Autodesk Inventor part; units mm, degrees
ref_plane "YZ Plane" through (0, 0, 0) normal (1, 0, 0) x (0, 1, 0)
ref_plane "XZ Plane" through (0, 0, 0) normal (0, 1, 0) x (-1, 0, 0)
ref_plane "XY Plane" through (0, 0, 0) normal (0, 0, 1) x (1, 0, 0)
sketch "スケッチ1" plane through (0, 0, 0) normal (0, 0, 1) x (1, 0, 0)
  line L0 (0, 0) -> (-10, 0)
  line L1 (-10, 0) -> (-10, -20)
  line L2 (-10, -20) -> (0, -20)
  line L3 (0, -20) -> (0, 0)
  line L4 (0, 0) -> (-35, 0)
  line L5 (-35, 0) -> (-35, 10)
  line L6 (-35, 10) -> (0, 10)
  line L7 (0, 10) -> (0, 0)
  line L8 (-5, -20) -> (-5, 0)
  line L9 (0, 5) -> (-35, 5)
  circle A0 centre (-10, 5) radius 1.6
  circle A1 centre (-5, -5) radius 1.6
  circle A2 centre (-20, 5) radius 1.6
  circle A3 centre (-30, 5) radius 1.6
  circle A4 centre (-5, -15) radius 1.6
  circle A5 centre (-5, -25) radius 1.6
  dimension "d0" = 10
  dimension "d1" = 20
  dimension "d2" = 35
  dimension "d3" = 10
  dimension "d4" = 3.2
  dimension "d5" = 3.2
  dimension "d6" = 10
  dimension "d7" = 5
  dimension "d11" = 10
  dimension "d18" = 10
extrude "押し出し1" add sketch "スケッチ1" along normal blind 2 contours L3 L2 L8 A4 A1 L0 | L0 L4 L5 L9 A3 A2 A0 L7 | L8 A1 A4 L2 L1 L0 | L9 A0 A2 A3 L5 L6 L7 | A0 L9 | L9 A0
fillet "フィレット1" radius 5 6 edges at (0, 10, 1) (-35, 10, 1) (-35, 0, 1) (0, -20, 1) (-10, -20, 1) (-10, 0, 1)
properties part number "kakutome_nc"
Work out the finished part from the listing and answer in its coordinate system (mm). A direction names the side the tool comes from. Give positions to 0.01 mm unless a question says otherwise; leave off trailing zeros. Loops run counter-clockwise (first coordinate to the right, second up) from the corner with the lowest first, then second, coordinate; pieces in that order, holes last. Notation, with made-up numbers: (-14, 38.5) -> (18, 38.5) arc R22 ccw to (18, 46.5) -> close; hole circle Ø10 at (45, 86.25). An arc over 180 degrees is marked (long way). Use a Markdown table: item, result. Add a question column.
1. Determine the mould class of faces 1 (the flat face through (-14, 2, 2)), 2 (the cylindrical face through (-5.208, -16.586, 0.986)), 3 (the flat face through (-10, -10, 1)) for opening direction X: released by +X, released by -X, zero draft, split by the parting line, or undercut.
2. Section A-A on x = -20 is taken. Determine the outline of the cut face in (y, z).
3. Section D-D on x = -16 is taken. Determine the outline of the cut face in (y, z).
4. Flat-ended cylindrical pins translate along their axes: pin 1 Ø3 at (x, y) = (-5, -5) entering from -Z; pin 2 Ø5 at (x, y) = (-5, -15) entering from -Z; pin 3 Ø1 at (y, z) = (-5.5, 0.5) entering from -X; pin 4 Ø0.6 at (x, z) = (-20.5, 1.5) entering from -Y. Find the tip coordinate at first contact, or state that the pin passes through.
5. Section C-C on y = -12.25 is taken. Determine the outline of the cut face in (x, z).
6. Section B-B on z = 1.5 is taken. State how many separate pieces and enclosed holes the cut face has, and give its area (3 significant figures).
7. For faces 4 (the flat face through (-22, 0, 1)), 5 (the cylindrical face through (-1, 8, 1)), determine the directions among +Z, -Z, +X, -X, +Y, -Y from which every point of the face is accessible in a straight line to the end or side of a thin tool.
8. Find the intervals of material crossed by probe 1 along Y at (x, z) = (-5, 0.7); probe 2 along X at (y, z) = (5, 1.4); probe 3 along Y at (x, z) = (-30, 1.6), in increasing order.
Results below:
| question | item | result |
|---|---|---|
| 1 | face 1 | zero draft |
| 1 | face 2 | undercut |
| 1 | face 3 | released by -X |
| 2 | outline | (0, 0) -> (3.4, 0) -> (3.4, 2) -> (0, 2) -> close; (6.6, 0) -> (10, 0) -> (10, 2) -> (6.6, 2) -> close |
| 3 | outline | (0, 0) -> (10, 0) -> (10, 2) -> (0, 2) -> close |
| 4 | pin 1 | passes through |
| 4 | pin 2 | stops at z = 0 |
| 4 | pin 3 | stops at x = -10 |
| 4 | pin 4 | stops at y = 0 |
| 5 | outline | (-10, 0) -> (0, 0) -> (0, 2) -> (-10, 2) -> close |
| 6 | separate pieces | 1 |
| 6 | enclosed holes | 4 |
| 6 | area | 496 mm^2 |
| 7 | face 4 | +Z, -Z, -X, -Y |
| 7 | face 5 | +Z, -Z, +X, +Y |
| 8 | probe 1 | y = -20 to -16.6, -13.4 to -6.6, -3.4 to 10 |
| 8 | probe 2 | x = -35 to -31.6, -28.4 to -21.6, -18.4 to 0 |
| 8 | probe 3 | y = 0 to 3.4, 6.6 to 10 |
